from build123d import *

# Parameters (mm, degrees)
F0_W      = 63
F0_H      = 70
F1_DEPTH  = 25
F3_DEPTH  = 63.001
F4_W      = 40
F4_H      = 10
F5_DEPTH  = 14
F7_DEPTH  = 40.001
F8_DEPTH  = 2
F9_R      = 8
F10_DEPTH = 2
F11_R     = 12


with BuildPart() as f1:
    # F0 (on Front) → F1 (new body)
    with BuildSketch(Plane.XZ):
        Rectangle(F0_W, F0_H)
    extrude(amount=F1_DEPTH)

    # F2 (on face) → F3 (cut, through all)
    with BuildSketch(Plane(origin=(-31.5, 0, 0), x_dir=(0, -1, 0), z_dir=(-1, 0, 0))):
        with BuildLine():
            ThreePointArc((0, 8.5052742394), (10.5828714835, 8.3586246097), (15.9170941003, 17.5))
            ThreePointArc((15.9170941003, 17.5), (10.5828714835, 26.6413753903), (0, 26.4947257606))
            Line((0, 26.4947257606), (0, 8.5052742394))
        make_face()
        with BuildLine():
            ThreePointArc((15.9170941003, -17.5), (10.5828714835, -8.3586246097), (0, -8.5052742394))
            Line((0, -8.5052742394), (0, -26.4947257606))
            ThreePointArc((0, -26.4947257606), (10.5828714835, -26.6413753903), (15.9170941003, -17.5))
        make_face()
    extrude(amount=-F3_DEPTH, mode=Mode.SUBTRACT)

    # F4 (on face) → F5 (join)
    with BuildSketch(Plane.XZ.offset(25)):
        Rectangle(F4_W, F4_H)
    extrude(amount=F5_DEPTH)

    # F6 (on face) → F7 (cut, through all)
    with BuildSketch(Plane(origin=(0, 0, -5), x_dir=(1, 0, 0), z_dir=(0, 0, -1))):
        with BuildLine():
            ThreePointArc((-6, 39), (0, 33), (6, 39))
            Line((6, 39), (-6, 39))
        make_face()
    extrude(amount=-F7_DEPTH, mode=Mode.SUBTRACT)

    # F6 (on face) → F8 (cut)
    with BuildSketch(Plane(origin=(0, 0, -5), x_dir=(1, 0, 0), z_dir=(0, 0, -1))):
        with BuildLine():
            ThreePointArc((-8, 39), (0, 31), (8, 39))
            Line((8, 39), (6, 39))
            ThreePointArc((6, 39), (0, 33), (-6, 39))
            Line((-6, 39), (-8, 39))
        make_face()
    extrude(amount=-F8_DEPTH, mode=Mode.SUBTRACT)

    # F9 (on face) → F10 (cut)
    with BuildSketch(Plane.XY.offset(5)):
        with Locations((0, -39)):
            Circle(F9_R)
    extrude(amount=-F10_DEPTH, mode=Mode.SUBTRACT)

    # F11
    f11_edges = [f1.edges().sort_by_distance(p)[0] for p in [
        (0, -25, 35),
        (0, -25, -35),
    ]]
    fillet(f11_edges, radius=F11_R)


solid = f1.part
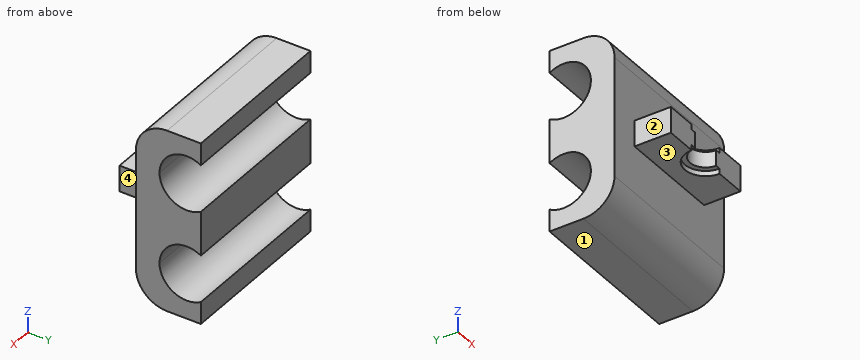
Verification items for the finished model (mm, model axes). Face numbers are marked on the shaded views. A direction names the side the tool comes from. Round coordinates to 2 decimals unless told otherwise and drop trailing zeros. Loops run counter-clockwise (first coordinate to the right, second up) from the corner with the lowest first, then second, coordinate; pieces in that order, holes last. Notation, with made-up numbers: (50, 17.5) - (63, 17.5) arc R10 cw to (63, 25.5) - close; hole circle Ø8 at (-24, -19). An arc over 180 degrees is marked (long way). Use one line per item in the form item = value.
1. Access from +Z, -Z, +X, -X, +Y, -Y to the whole of each face (thin tool, end or side, straight path). Record for the marked faces 1, 2, 3 and 4.
A:
face_1 = -Z, +X, -X, +Y, -Y
face_2 = +Z, -Z, -X, -Y
face_3 = -Z, +X, -X, -Y
face_4 = +Z, -Z, +X, -Y
2. Section check D-D on x = -14.5. Record the cut outline in (y, z), and give its area (3 significant figures).
A:
outline = (-39, -5) - (-25, -5) - (-25, -23) arc R12 ccw to (-13, -35) - (0, -35) - (0, -26.49) arc R10.5 cw (long way) to (0, -8.51) - (0, 8.51) arc R10.5 cw (long way) to (0, 26.49) - (0, 35) - (-13, 35) arc R12 ccw to (-25, 23) - (-25, 5) - (-39, 5) - close
area = 1,260 mm²
3. Scan lines: probe 1 along Z at (x, y) = (-19, -5); probe 2 along Y at (x, z) = (-8, 6.5); probe 3 along Z at (x, y) = (-6, -7). Record each from-to range of solid material in increasing order.
A:
probe_1 = -35 to -27.99, -7.01 to 7.01, 27.99 to 35
probe_2 = -25 to 0
probe_3 = -35 to -27.88, -7.12 to 7.12, 27.88 to 35
4. Section check B-B on y = -7.5. Record the cut outline in (x, z), and give its area (3 significant figures).
A:
outline = (-31.5, -35) - (31.5, -35) - (31.5, -27.79) - (-31.5, -27.79) - close; (-31.5, -7.21) - (31.5, -7.21) - (31.5, 7.21) - (-31.5, 7.21) - close; (-31.5, 27.79) - (31.5, 27.79) - (31.5, 35) - (-31.5, 35) - close
area = 1,820 mm²
5. Section check C-C on y = -26. Record the cut outline in (x, z).
A:
outline = (-20, -5) - (20, -5) - (20, 5) - (-20, 5) - close
6. Section check A-A on x = -22. Record the cut outline in (y, z), and give its area (3 significant figures).
A:
outline = (-25, -23) arc R12 ccw to (-13, -35) - (0, -35) - (0, -26.49) arc R10.5 cw (long way) to (0, -8.51) - (0, 8.51) arc R10.5 cw (long way) to (0, 26.49) - (0, 35) - (-13, 35) arc R12 ccw to (-25, 23) - close
area = 1,120 mm²
7. Gauge pin test, flat ends, axial feed: pin 1 Ø2.5 at (x, y) = (-1, -35) entering from +Z (1 decimal); pin 2 Ø10 at (x, y) = (19, -24) entering from +Z; pin 3 Ø4 at (x, y) = (6, -34.5) entering from +Z; pin 4 Ø9 at (x, y) = (-2.5, -36) entering from -Z. Record the tip position at first contact, or that the pin passes through.
A:
pin_1 = through
pin_2 = 33.39
pin_3 = 5
pin_4 = -5
